```python
from build123d import *

# Parameters (mm, degrees)
RESSALTO_EXTRUS_O1_DEPTH      = 30
RESSALTO_EXTRUS_O1_DEPTH_BACK = 30
ESBO_O1_R                     = 7.5
ESBO_O2_W                     = 52
ESBO_O2_H                     = 143.285030211
CORTE_EXTRUS_O1_DEPTH         = 123.474851541
CHANFRO1_SIZE                 = 5
ESBO_O3_R                     = 8.5
RESSALTO_EXTRUS_O2_DEPTH      = 100


with BuildPart() as part:
    # Esbo_o1 → Ressalto-extrus_o1 (new, two sides: drawn at the far end of the back side and taken through both)
    with BuildSketch(Plane(origin=(0, 0, 0), x_dir=(0, 0, -1), z_dir=(1, 0, 0)).offset(-RESSALTO_EXTRUS_O1_DEPTH_BACK)):
        with BuildLine():
            Line((17.662425064, 66.241666463), (17.662425064, 96.241666463))
            Line((17.662425064, 96.241666463), (57.662425064, 96.241666463))
            Line((57.662425064, 96.241666463), (57.662425064, 66.241666463))
            Line((57.662425064, 66.241666463), (25.862440111, -52.968524997))
            ThreePointArc((25.862440111, -52.968524997), (-1.100846101, -61.511428289), (-9.643749393, -34.548142078))
            Line((-9.643749393, -34.548142078), (17.662425064, 66.241666463))
        make_face()
        with Locations((8.109345359, -43.758333537)):
            Circle(ESBO_O1_R, mode=Mode.SUBTRACT)
    extrude(amount=RESSALTO_EXTRUS_O1_DEPTH + RESSALTO_EXTRUS_O1_DEPTH_BACK)

    # Esbo_o2 → Corte-extrus_o1 (cut, through all)
    with BuildSketch(Plane(origin=(0, 0, -57.662425064), x_dir=(-1, 0, 0), z_dir=(0, 0, -1))):
        with Locations((0, -5.400848643)):
            Rectangle(ESBO_O2_W, ESBO_O2_H)
    extrude(amount=-CORTE_EXTRUS_O1_DEPTH, mode=Mode.SUBTRACT)

    # Chanfro1
    chanfro1_edges = [part.edges().sort_by_distance(p)[0] for p in [
        (0, 96.241666463, -17.662425064),
        (0, 96.241666463, -57.662425064),
        (-30, 96.241666463, -37.662425064),
        (30, 96.241666463, -37.662425064),
    ]]
    chamfer(chanfro1_edges, length=CHANFRO1_SIZE)

    # Esbo_o3 → Ressalto-extrus_o2 (add)
    with BuildSketch(Plane(origin=(0, 96.241666463, 0), x_dir=(1, 0, 0), z_dir=(0, 1, 0))):
        with Locations(Location((0, 37.662425064, 0), (0, 0, 270))):
            Circle(ESBO_O3_R)
    extrude(amount=RESSALTO_EXTRUS_O2_DEPTH)


solid = part.part
```
Geometry check sheet. Reference: the model listing, model coordinates, mm. A direction names the side the tool comes from. Round coordinates to 2 decimals unless told otherwise and drop trailing zeros. Order: outer loops, then holes, each group sorted by start corner. A loop starts at its lowest first (then second) coordinate and runs counter-clockwise, first axis right, second up. Notation, with made-up numbers: (-32, 81) - (-8, 81) arc R13 cw to (-8, 92) - close; hole circle Ø2 at (47.25, -14.5). An arc over 180 degrees is marked (long way). Use a Markdown table: item, result. Add a question column.
(1) Depth check by flat-ended pin: pin 1 (1.5 mm diameter, centred on y = 127, z = -44.5, fed in from -X); pin 2 (20 mm diameter, centred on x = 10, z = -36.5, fed in from -Y); pin 3 (12.5 mm diameter, centred on x = -11, y = 79.5, fed in from +Z); pin 4 (10 mm diameter, centred on x = -18.5, z = 4, fed in from -Y). Enter the tip coordinate at first touch or a pass-through.
(2) Release check for a two-part mould opening along Z. For faces 4 (the cylindrical face through (27.97, -51.08, -6.48)), 5 (the flat face through (-28.028, 15.141, -3.818)), 6 (the flat face through (0, 66.242, -38)) record: pulls with the +Z half, pulls with the -Z half, needs draft (parallel to the pull), parting line crosses it, or undercut.
(3) Tool access check on faces 1 (the flat face through (0, 79, -57.662)), 2 (the flat face through (26, 0, -23)), 3 (the flat face through (0, 79, -17.662)). Record the directions out of +Z, -Z, +X, -X, +Y, -Y that give a thin tool (end or side, any length) a straight path to the whole face; none if there is none.
(4) Material ranges on line 1 along X through (y, z) = (-4.5, -37); line 2 along Y through (x, z) = (19.5, -31.5); line 3 along Z through (x, y) = (1, 87.5), recorded low to high. Write a range as [from, to].
(5) Sectioned sample at B-B, the plane x = 17. Enter the section's corners in (y, z), and give its area (4 significant figures).
(6) Sectioned sample at C-C, the plane z = -42.5. Enter the section's corners in (x, y), and give its area (3 significant figures).
(7) Sectioned sample at D-D, the plane x = 0. Enter the section's corners in (y, z), and give its area (4 significant figures).
(8) Sectioned sample at A-A, the plane y = 52. Enter the section's corners in (x, z).
Answers below:
| question | item | result |
|---|---|---|
| 1 | pin 1 | x = -5.93 |
| 1 | pin 2 | y = 66.24 |
| 1 | pin 3 | z = -17.66 |
| 1 | pin 4 | through |
| 2 | face 4 | undercut |
| 2 | face 5 | pulls with the +Z half |
| 2 | face 6 | needs draft |
| 3 | face 1 | -Z, +X, -X, +Y, -Y |
| 3 | face 2 | +Z, -Z, -Y |
| 3 | face 3 | +Z, +X, -X, +Y |
| 4 | line 1 | [-30, -26], [26, 30] |
| 4 | line 2 | [66.24, 96.24] |
| 4 | line 3 | [-57.66, -17.66] |
| 5 | outline | (66.24, -57.66) - (91.24, -57.66) - (96.24, -52.66) - (96.24, -22.66) - (91.24, -17.66) - (66.24, -17.66) - close |
| 5 | area | 1,175 mm² |
| 6 | outline | (-30, 9.4) - (-26, 9.4) - (-26, 66.24) - (26, 66.24) - (26, 9.4) - (30, 9.4) - (30, 91.24) - (25, 96.24) - (6.99, 96.24) - (6.99, 196.24) - (-6.99, 196.24) - (-6.99, 96.24) - (-25, 96.24) - (-30, 91.24) - close |
| 6 | area | 3,630 mm² |
| 7 | outline | (66.24, -57.66) - (91.24, -57.66) - (96.24, -52.66) - (96.24, -46.16) - (196.24, -46.16) - (196.24, -29.16) - (96.24, -29.16) - (96.24, -22.66) - (91.24, -17.66) - (66.24, -17.66) - close |
| 7 | area | 2,875 mm² |
| 8 | outline | (-30, -53.86) - (-26, -53.86) - (-26, -13.8) - (-30, -13.8) - close; (26, -53.86) - (30, -53.86) - (30, -13.8) - (26, -13.8) - close |
